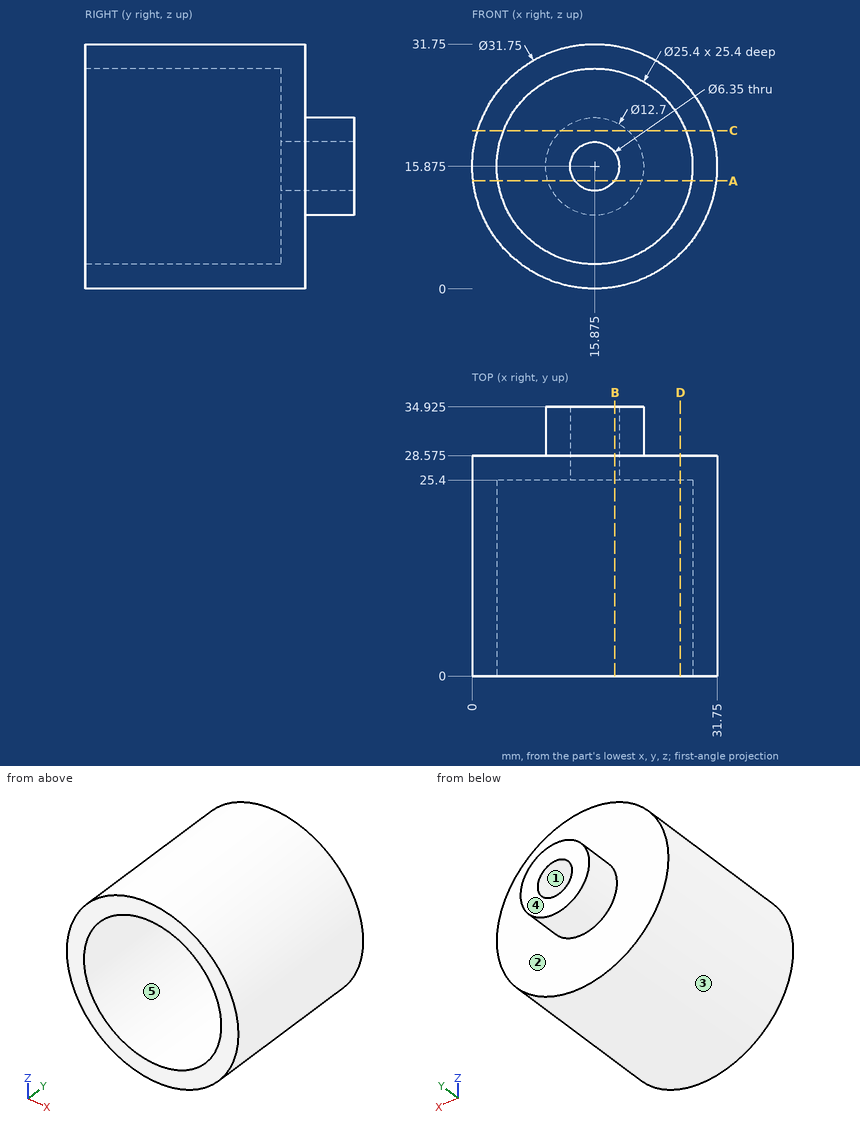
Can you work these out from the drawing? Everything is in mm from the part's minimum corner. A direction names the side the tool comes from. Round coordinates to 2 decimals unless told otherwise and drop trailing zeros. Order: outer loops, then holes, each group sorted by start corner. A loop starts at its lowest first (then second) coordinate and runs counter-clockwise, first axis right, second up. Notation, with made-up numbers: M 81,20 L 124,20 A22 cw 124,48 Z; hole C 9.5,-2 d7. An arc over 180 degrees is marked long. One line per question, with ' | ' between items.
1) For the marked faces 1 and 2, which set-ups out of +Z, -Z, +X, -X, +Y, -Y let a thin tool reach every point of the face, with its end or its side?
Working result:
face 1: +Y, -Y | face 2: +Y
2) I want a section at C-C, the plane z = 20.5. Write out the boundary of the cut face in (x, y) (3 decimals).
Working result:
outline: M 0.689,0 L 4.047,0 L 4.047,25.4 L 27.703,25.4 L 27.703,0 L 31.061,0 L 31.061,28.575 L 20.226,28.575 L 20.226,34.925 L 11.524,34.925 L 11.524,28.575 L 0.689,28.575 Z
3) I want a section at D-D, the plane x = 27. Write out the boundary of the cut face in (y, z) (3 decimals).
Working result:
outline: M 0,4.55 L 28.575,4.55 L 28.575,27.2 L 0,27.2 L 0,22.001 L 25.4,22.001 L 25.4,9.749 L 0,9.749 Z
4) If we mould it in two halves opening along Z, with no side actions, what happens to the marked faces 3, 4 and 5? For each: +Z half, -Z half, draft (parallel to the pull), parting line (faces both ways), or undercut.
Working result:
face 3: parting line | face 4: draft | face 5: undercut
5) For pin 1 Ø16 at (x, z) = (16.5, 8) entering from +Y (3 decimals); pin 2 Ø2 at (x, z) = (25.5, 5) entering from +Y (3 decimals); pin 3 Ø5 at (x, y) = (22.5, 17.5) entering from +Z; pin 4 Ø6 at (x, y) = (25, 22.5) entering from -Z, each with a flat end and sliding along its axis, tell me the tip position at first contact or that it passes through.
Working result:
pin 1: y = 34.925 | pin 2: y = 28.575 | pin 3: z = 31.2 | pin 4: z = 1.23
6) I want a section at A-A, the plane z = 14. Write out the boundary of the cut face in (x, y) (3 decimals).
Working result:
outline: M 0.111,0 L 3.314,0 L 3.314,25.4 L 13.313,25.4 L 13.313,34.925 L 9.808,34.925 L 9.808,28.575 L 0.111,28.575 Z; M 18.437,25.4 L 28.436,25.4 L 28.436,0 L 31.639,0 L 31.639,28.575 L 21.942,28.575 L 21.942,34.925 L 18.437,34.925 Z
7) I need wall thicknesses on line 1 along Y through (x, z) = (10.5, 9) (3 decimals); line 2 along Y through (x, z) = (11.5, 13) (3 decimals); line 3 along Z through (x, y) = (21, 11.5) (3 decimals). Which ranges of each line are inside material? Lowest first, please.
Working result:
line 1: 25.4 to 28.575 | line 2: 25.4 to 34.925 | line 3: 0.85 to 4.255, 27.495 to 30.9
8) I want a section at B-B, the plane x = 18.5. Write out the boundary of the cut face in (y, z) (3 decimals).
Working result:
outline: M 0,0.219 L 28.575,0.219 L 28.575,10.093 L 34.925,10.093 L 34.925,14.089 L 25.4,14.089 L 25.4,3.449 L 0,3.449 Z; M 0,28.301 L 25.4,28.301 L 25.4,17.661 L 34.925,17.661 L 34.925,21.657 L 28.575,21.657 L 28.575,31.531 L 0,31.531 Z
